Study the drawing (mm; zero at the part's minimum x, y, z) and answer. Coordinates: 2 decimals unless noted, no trailing zeros. Loops run counter-clockwise (first coordinate to the right, second up) from the corner with the lowest first, then second, coordinate; pieces in that order, holes last. Notation, with made-up numbers: (81.5, 18.5) -> (131.5, 18.5) arc R20 cw to (131.5, 25.5) -> close; hole circle Ø2 at (76.5, 79). An arc over 180 degrees is marked (long way). Answer as a JSON object with one key per item and string values. Group by question number.
Q1. The part is cut by section A-A on y = 75. Write down the section's boundary in (x, z), and give its area (3 significant figures).
Q2. The part is cut by section D-D on z = 2.5. Write down the section's boundary in (x, y).
Q3. Determine the mould class of the marked faces 1, 2 and 3 for opening direction X: released by +X, released by -X, zero draft, split by the parting line, or undercut.
Q4. The part is cut by section C-C on x = 20. Write down the section's boundary in (y, z).
Q5. Straight lines are drawn through the part: line 1 along Y through (x, z) = (75, 3.25); line 2 along Y through (x, z) = (17.5, 5.5); line 3 along X through (y, z) = (133, 8.25). For each, find the intervals that lie inside material, in ascending order. Write a range as [from, to].
Q6. Each of these flat-tipped pins is pushed along its axis until it touches: P1, Ø5, axis at x = 36.5, z = 7.5, coming from the +Y side; P2, Ø6, axis at x = 67.5, z = 6.5, coming from the +Y side; P3, Ø6, axis at y = 129, z = 9, coming from the -X side. Where does it stop, or does it pass through?
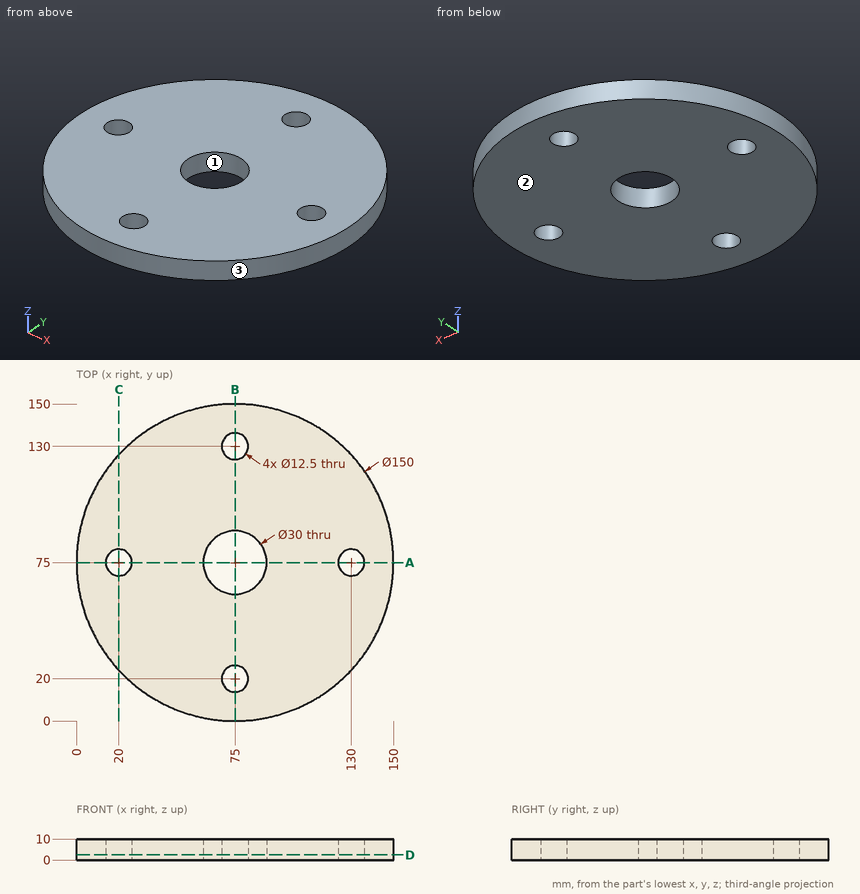
Final values:
{
 "1": {"outline": "(0, 0) -> (13.75, 0) -> (13.75, 10) -> (0, 10) -> close; (26.25, 0) -> (60, 0) -> (60, 10) -> (26.25, 10) -> close; (90, 0) -> (123.75, 0) -> (123.75, 10) -> (90, 10) -> close; (136.25, 0) -> (150, 0) -> (150, 10) -> (136.25, 10) -> close", "area": "950 mm2"},
 "2": {"outline": "circle Ø150 at (75, 75); hole circle Ø12.5 at (20, 75); hole circle Ø30 at (75, 75); hole circle Ø12.5 at (75, 20); hole circle Ø12.5 at (75, 130); hole circle Ø12.5 at (130, 75)"},
 "3": {"face 1": "undercut", "face 2": "zero draft", "face 3": "split by the parting line"},
 "4": {"outline": "(24.01, 0) -> (68.75, 0) -> (68.75, 10) -> (24.01, 10) -> close; (81.25, 0) -> (125.99, 0) -> (125.99, 10) -> (81.25, 10) -> close"},
 "5": {"line 1": "y = [0, 13.75], [26.25, 60], [90, 123.75], [136.25, 150]", "line 2": "y = [26.85, 69.27], [80.73, 123.15]", "line 3": "x = [27.45, 69.52], [80.48, 122.55]"},
 "6": {"P1": "stops at y = 140.8", "P2": "stops at y = 149.86", "P3": "stops at x = 20.01"}
}
